Input: part model. Units: mm. Frame: model coordinates. Face numbers are marked on the shaded views. A direction names the side the tool comes from. Round coordinates to 2 decimals unless told otherwise and drop trailing zeros. Loops run counter-clockwise (first coordinate to the right, second up) from the corner with the lowest first, then second, coordinate; pieces in that order, holes last. Notation, with made-up numbers: M -35.5,-8.5 L -19.5,-8.5 A19 ccw -19.5,14.5 Z; hole C 6.25,43 d1. An arc over 180 degrees is marked long. Use one line per item in the form item = value. Start each with the question number.
Q1. Ray query, line 1 along X through (y, z) = (-21, 49.5); line 2 along Y through (x, z) = (-23, 48). Return the intervals inside material, ascending.
Q2. First-contact query: P1, Ø6, axis at x = 18.5, z = 44, coming from the +Y side; P2, Ø12, axis at x = -2, z = 56.5, coming from the +Y side; P3, Ø1.5, axis at y = 15, z = 41.5, coming from the -X side; P4, Ø5.5, axis at x = -23.5, y = 23.5, coming from the +Z side. Flat tips, straight axial feed; report the tip coordinate or a pass-through.
Q3. Section query B-B, the plane y = -12. Output: boundary loops of the cut face in (x, z), and give its area (3 significant figures).
Q4. Section query A-A, the plane x = 7. Output: boundary loops of the cut face in (y, z).
Q5. Mould query, pull axis Z, two halves, no side actions, for the marked faces 4, 5 and 6. Classes: pulls with the +Z half, pulls with the -Z half, needs draft (parallel to the pull), parting line crosses it, or undercut.
Q6. Section query C-C, the plane z = 11. Output: boundary loops of the cut face in (x, y), and give its area (3 significant figures).
Q7. Access query for the marked faces 1, 2 and 3. Directions: +Z, -Z, +X, -X, +Y, -Y. A direction counts if a zero-diameter tool reaches every point of the face in a straight line with its end or side. Return the directions, or none.
Q8. Section query D-D, the plane z = 24. Output: boundary loops of the cut face in (x, y), and give its area (3 significant figures).
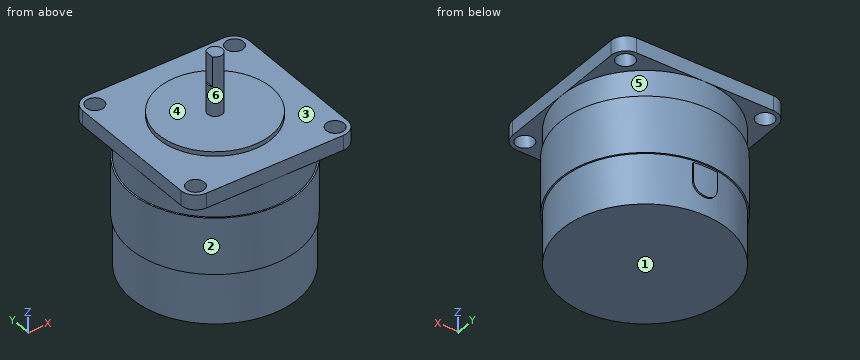
```python
from build123d import *

# Parameters (mm, degrees)
SKETCH1_R           = 28
EXTRUDE1_DEPTH      = 45
SKETCH2_W           = 56
SKETCH2_H           = 56
EXTRUDE2_DEPTH      = 5
SKETCH4_R           = 3
EXTRUDE3_DEPTH      = 5
SKETCH5_W           = 0.5
SKETCH5_H           = 19
SKETCH7_R           = 19
EXTRUDE4_DEPTH      = 1.5
SKETCH9_R           = 2.5
EXTRUDE5_DEPTH      = 20
SKETCH10_W          = 5
SKETCH10_H          = 3
EXTRUDE6_DEPTH      = 10
FILLET1_R           = 5
EXTRUDE7_REACH      = 84.078
EXTRUDE7_END_RADIUS = 28.5


with BuildPart() as part:
    # Sketch1 → Extrude1 (new body)
    with BuildSketch(Plane.XY):
        Circle(SKETCH1_R)
    extrude(amount=EXTRUDE1_DEPTH)

    # Sketch2 → Extrude2 (add)
    with BuildSketch(Plane.XY.offset(45)):
        Rectangle(SKETCH2_W, SKETCH2_H)
    extrude(amount=EXTRUDE2_DEPTH)

    # Sketch4 → Extrude3 (cut)
    with BuildSketch(Plane.XY.offset(50)):
        with Locations((-23.5, 23.5)):
            Circle(SKETCH4_R)
        with Locations((23.5, 23.5)):
            Circle(SKETCH4_R)
        with Locations((-23.5, -23.5)):
            Circle(SKETCH4_R)
        with Locations((23.5, -23.5)):
            Circle(SKETCH4_R)
    extrude(amount=-EXTRUDE3_DEPTH, mode=Mode.SUBTRACT)

    # Sketch5 → Revolve2 (revolve)
    with BuildSketch(Plane(origin=(0, 0, 0), x_dir=(1, 0, 0), z_dir=(0, 1, 0)), mode=Mode.PRIVATE) as revolve2_sk:
        with Locations((28.25, -26.5)):
            Rectangle(SKETCH5_W, SKETCH5_H)
    revolve(revolve2_sk.sketch.rotate(Axis((0, 0, 0), (0, 0, 1)), 180), axis=Axis((0, 0, 0), (0, 0, 1)))

    # Sketch7 → Extrude4 (add)
    with BuildSketch(Plane.XY.offset(50)):
        Circle(SKETCH7_R)
    extrude(amount=EXTRUDE4_DEPTH)

    # Sketch9 → Extrude5 (add)
    with BuildSketch(Plane.XY.offset(51.5)):
        Circle(SKETCH9_R)
    extrude(amount=EXTRUDE5_DEPTH)

    # Sketch10 → Extrude6 (cut)
    with BuildSketch(Plane.XY.offset(71.5)):
        with Locations((-4.5, 0)):
            Rectangle(SKETCH10_W, SKETCH10_H)
    extrude(amount=-EXTRUDE6_DEPTH, mode=Mode.SUBTRACT)

    # Fillet1
    fillet1_edges = [part.edges().sort_by_distance(p)[0] for p in [
        (28, -28, 47.5),
        (28, 28, 47.5),
        (-28, 28, 47.5),
        (-28, -28, 47.5),
    ]]
    fillet(fillet1_edges, radius=FILLET1_R)

    # Extrude7: up to this cylinder (the profile starts inside it)
    extrude7_end = Plane(origin=(0, 0, 11.385608), z_dir=(0, 0, -1)) * Cylinder(EXTRUDE7_END_RADIUS, 226.156, mode=Mode.PRIVATE)
    # Sketch11 → Extrude7 (add, up to the surface)
    with BuildSketch(Plane(origin=(0, 0, 0), x_dir=(1, 0, 0), z_dir=(0, 1, 0)), mode=Mode.PRIVATE) as extrude7_sk1:
        with BuildLine():
            Line((-4, -16), (4, -16))
            Line((4, -16), (4, -10))
            ThreePointArc((4, -10), (0, -6), (-4, -10))
            Line((-4, -10), (-4, -16))
        make_face()
    extrude7_tool1 = extrude(extrude7_sk1.sketch, amount=EXTRUDE7_REACH, mode=Mode.PRIVATE) & extrude7_end
    add(extrude7_tool1.solids().sort_by_distance((0, 0, 11.385608))[0])


solid = part.part
```
Results found:
q1.line_1 = -28 to -25.16, -21.84 to 21.84, 25.16 to 28
q1.line_2 = -28 to -26.46, -20.54 to 20.54, 26.46 to 28
q2.P1 = 28
q2.P2 = 19
q2.P3 = -24.1
q2.P4 = through
q3.outline = M -28,45 L -25.3,45 L -25.3,36 L -25.85,36 L -25.85,17 L -25.3,17 L -25.3,0 L 25.3,0 L 25.3,17 L 25.85,17 L 25.85,36 L 25.3,36 L 25.3,45 L 28,45 L 28,50 L 14.73,50 L 14.73,51.5 L -14.73,51.5 L -14.73,50 L -28,50 Z
q3.area = 2,620 mm²
q4.outline = M -28,45 L -27.11,45 L -27.11,36 L -27.63,36 L -27.63,17 L -27.11,17 L -27.11,0 L 27.11,0 L 27.11,17 L 27.63,17 L 27.63,36 L 27.11,36 L 27.11,45 L 28,45 L 28,50 L 17.66,50 L 17.66,51.5 L -17.66,51.5 L -17.66,50 L -28,50 Z
q5.face_4 = pulls with the +Z half
q5.face_5 = undercut
q5.face_6 = needs draft
q6.outline = M -4,27.71 A28 ccw long 4,27.71 L 4,28.22 A28.5 ccw -4,28.22 Z
q6.area = 2,470 mm²
q7.face_1 = -Z, +X, -X, +Y, -Y
q7.face_2 = -Z
q7.face_3 = +Z
q8.outline = C 0,0 d57
q8.area = 2,550 mm²
